Design review of the part built by this model. Coordinates are the model's own, in mm. Give positions to 0.01 mm unless a question says otherwise; leave off trailing zeros. Write each loop counter-clockwise with the first axis right and the second up, starting at its lowest first coordinate (ties: lowest second). Pieces come first, ordered by that corner, then holes. Notation, with made-up numbers: M 40,41.5 L 70,41.5 A20 ccw 70,61.5 Z; hole C 67,2 d9. An arc over 180 degrees is marked long. Use one line per item in the form item = value. Start each with the question number.
from build123d import *

# Parameters (mm, degrees)
SKETCH1_W           = 110
SKETCH1_H           = 85
BOSS_EXTRUDE1_DEPTH = 3
BOSS_EXTRUDE2_DEPTH = 1
SKETCH3_R           = 2.6
SKETCH3_R_2         = 1.5
CUT_EXTRUDE1_DEPTH  = 1
CUT_EXTRUDE2_REACH  = 6
SKETCH3_2_R         = 1.5
FILLET1_R           = 3
SKETCH15_R          = 1.75
CUT_EXTRUDE3_REACH  = 6
SKETCH17_R          = 3
SKETCH17_3_R        = 6
SKETCH17_3_R_2      = 3
CUT_EXTRUDE4_DEPTH  = 2
SKETCH18_W          = 20.4
SKETCH18_H          = 31.7
CUT_EXTRUDE5_DEPTH  = 5
SKETCH18_4_W        = 17
SKETCH18_4_H        = 5.15
BOSS_EXTRUDE3_DEPTH = 1.5
SKETCH19_R          = 1
CUT_EXTRUDE6_DEPTH  = 5
FILLET2_R           = 1


with BuildPart() as part:
    # Sketch1 → Boss-Extrude1 (new body)
    with BuildSketch(Plane(origin=(0, 0, 0), x_dir=(1, 0, 0), z_dir=(0, 1, 0))):
        with Locations((55, 42.5)):
            Rectangle(SKETCH1_W, SKETCH1_H)
    extrude(amount=BOSS_EXTRUDE1_DEPTH)

    # Sketch2 → Boss-Extrude2 (add)
    with BuildSketch(Plane.XZ):
        with BuildLine():
            ThreePointArc((100.9, -79.9), (102.071572875, -77.071572875), (104.9, -75.9))
            Line((104.9, -75.9), (104.9, -9.1))
            ThreePointArc((104.9, -9.1), (102.071572875, -7.928427125), (100.9, -5.1))
            Line((100.9, -5.1), (9.1, -5.1))
            ThreePointArc((9.1, -5.1), (7.928427125, -7.928427125), (5.1, -9.1))
            Line((5.1, -9.1), (5.1, -75.9))
            ThreePointArc((5.1, -75.9), (7.928427125, -77.071572875), (9.1, -79.9))
            Line((9.1, -79.9), (100.9, -79.9))
        make_face()
    extrude(amount=BOSS_EXTRUDE2_DEPTH)

    # Sketch3 → Cut-Extrude1 (cut)
    with BuildSketch(Plane(origin=(0, 3, 0), x_dir=(1, 0, 0), z_dir=(0, 1, 0))):
        with Locations((4, 81)):
            Circle(SKETCH3_R)
        with Locations((4, 81)):
            Circle(SKETCH3_R_2, mode=Mode.SUBTRACT)
        with Locations((106, 81)):
            Circle(SKETCH3_R)
        with Locations((106, 81)):
            Circle(SKETCH3_R_2, mode=Mode.SUBTRACT)
        with Locations((106, 4)):
            Circle(SKETCH3_R)
        with Locations((106, 4)):
            Circle(SKETCH3_R_2, mode=Mode.SUBTRACT)
        with Locations((4, 4)):
            Circle(SKETCH3_R)
        with Locations((4, 4)):
            Circle(SKETCH3_R_2, mode=Mode.SUBTRACT)
    extrude(amount=-CUT_EXTRUDE1_DEPTH, mode=Mode.SUBTRACT)

    # Sketch3<2> → Cut-Extrude2 (cut, up to next)
    with BuildSketch(Plane(origin=(0, 3, 0), x_dir=(1, 0, 0), z_dir=(0, 1, 0)), mode=Mode.PRIVATE) as cut_extrude2_sk1:
        with Locations((4, 81)):
            Circle(SKETCH3_2_R)
    cut_extrude2_tool1 = extrude(cut_extrude2_sk1.sketch, amount=-CUT_EXTRUDE2_REACH, mode=Mode.PRIVATE) & part.part
    add(cut_extrude2_tool1.solids().sort_by_distance((4, 3, -81))[0], mode=Mode.SUBTRACT)
    # Sketch3<2> → Cut-Extrude2 (cut, up to next)
    with BuildSketch(Plane(origin=(0, 3, 0), x_dir=(1, 0, 0), z_dir=(0, 1, 0)), mode=Mode.PRIVATE) as cut_extrude2_sk2:
        with Locations((106, 81)):
            Circle(SKETCH3_2_R)
    cut_extrude2_tool2 = extrude(cut_extrude2_sk2.sketch, amount=-CUT_EXTRUDE2_REACH, mode=Mode.PRIVATE) & part.part
    add(cut_extrude2_tool2.solids().sort_by_distance((106, 3, -81))[0], mode=Mode.SUBTRACT)
    # Sketch3<2> → Cut-Extrude2 (cut, up to next)
    with BuildSketch(Plane(origin=(0, 3, 0), x_dir=(1, 0, 0), z_dir=(0, 1, 0)), mode=Mode.PRIVATE) as cut_extrude2_sk3:
        with Locations((106, 4)):
            Circle(SKETCH3_2_R)
    cut_extrude2_tool3 = extrude(cut_extrude2_sk3.sketch, amount=-CUT_EXTRUDE2_REACH, mode=Mode.PRIVATE) & part.part
    add(cut_extrude2_tool3.solids().sort_by_distance((106, 3, -4))[0], mode=Mode.SUBTRACT)
    # Sketch3<2> → Cut-Extrude2 (cut, up to next)
    with BuildSketch(Plane(origin=(0, 3, 0), x_dir=(1, 0, 0), z_dir=(0, 1, 0)), mode=Mode.PRIVATE) as cut_extrude2_sk4:
        with Locations((4, 4)):
            Circle(SKETCH3_2_R)
    cut_extrude2_tool4 = extrude(cut_extrude2_sk4.sketch, amount=-CUT_EXTRUDE2_REACH, mode=Mode.PRIVATE) & part.part
    add(cut_extrude2_tool4.solids().sort_by_distance((4, 3, -4))[0], mode=Mode.SUBTRACT)

    # Fillet1
    fillet1_edges = [part.edges().sort_by_distance(p)[0] for p in [
        (0, 1.5, -85),
        (110, 1.5, -85),
        (110, 1.5, 0),
        (0, 1.5, 0),
    ]]
    fillet(fillet1_edges, radius=FILLET1_R)

    # Cut-Sweep3: sweep along a path in Sketch14
    with BuildLine(Plane.XZ) as cut_sweep3_path:
        Line((7.35, -5.1), (7.35, -3.35))
        Line((7.35, -3.35), (102.65, -3.35))
        Line((102.65, -3.35), (102.65, -5.1))
        ThreePointArc((102.65, -5.1), (103.309009742, -6.690990258), (104.9, -7.35))
        Line((104.9, -7.35), (106.65, -7.35))
        Line((106.65, -7.35), (106.65, -77.65))
        Line((106.65, -77.65), (104.9, -77.65))
        ThreePointArc((104.9, -77.65), (103.309009742, -78.309009742), (102.65, -79.9))
        Line((102.65, -79.9), (102.65, -81.65))
        Line((102.65, -81.65), (7.35, -81.65))
        Line((7.35, -81.65), (7.35, -79.9))
        ThreePointArc((7.35, -79.9), (6.690990258, -78.309009742), (5.1, -77.65))
        Line((5.1, -77.65), (3.35, -77.65))
        Line((3.35, -77.65), (3.35, -7.35))
        Line((3.35, -7.35), (5.1, -7.35))
        ThreePointArc((5.1, -7.35), (6.690990258, -6.690990258), (7.35, -5.1))
    # Sketch15 → Cut-Sweep3 (sweep, cut)
    with BuildSketch(Plane.XY.offset(-77.65)):
        with Locations((106.65, 0)):
            Circle(SKETCH15_R)
    sweep(path=cut_sweep3_path.line, transition=Transition.RIGHT, mode=Mode.SUBTRACT)

    # Sketch17 → Cut-Extrude3 (cut, up to next)
    with BuildSketch(Plane.XZ.offset(1), mode=Mode.PRIVATE) as cut_extrude3_sk1:
        with Locations((20, -20.1)):
            Circle(SKETCH17_R)
    cut_extrude3_tool1 = extrude(cut_extrude3_sk1.sketch, amount=-CUT_EXTRUDE3_REACH, mode=Mode.PRIVATE) & part.part
    add(cut_extrude3_tool1.solids().sort_by_distance((20, -1, -20.1))[0], mode=Mode.SUBTRACT)
    # Sketch17 → Cut-Extrude3 (cut, up to next)
    with BuildSketch(Plane.XZ.offset(1), mode=Mode.PRIVATE) as cut_extrude3_sk2:
        with Locations((90, -20.1)):
            Circle(SKETCH17_R)
    cut_extrude3_tool2 = extrude(cut_extrude3_sk2.sketch, amount=-CUT_EXTRUDE3_REACH, mode=Mode.PRIVATE) & part.part
    add(cut_extrude3_tool2.solids().sort_by_distance((90, -1, -20.1))[0], mode=Mode.SUBTRACT)

    # Sketch17<3> → Cut-Extrude4 (cut)
    with BuildSketch(Plane.XZ.offset(1)):
        with Locations((90, -20.1)):
            Circle(SKETCH17_3_R)
        with Locations((90, -20.1)):
            Circle(SKETCH17_3_R_2, mode=Mode.SUBTRACT)
        with Locations((20, -20.1)):
            Circle(SKETCH17_3_R)
        with Locations((20, -20.1)):
            Circle(SKETCH17_3_R_2, mode=Mode.SUBTRACT)
    extrude(amount=-CUT_EXTRUDE4_DEPTH, mode=Mode.SUBTRACT)

    # Sketch18 → Cut-Extrude5 (cut, through all)
    with BuildSketch(Plane.XZ.offset(1)):
        with Locations((55, -49.908642181)):
            Rectangle(SKETCH18_W, SKETCH18_H)
    extrude(amount=-CUT_EXTRUDE5_DEPTH, mode=Mode.SUBTRACT)

    # Sketch18<4> → Boss-Extrude3 (add)
    with BuildSketch(Plane.XZ.offset(1)):
        with Locations((55, -31.483642181)):
            Rectangle(SKETCH18_4_W, SKETCH18_4_H)
        with Locations((55, -68.333642181)):
            Rectangle(SKETCH18_4_W, SKETCH18_4_H)
    extrude(amount=BOSS_EXTRUDE3_DEPTH)

    # Sketch19 → Cut-Extrude6 (cut)
    with BuildSketch(Plane.XZ.offset(2.5)):
        with Locations((55, -31.908642181)):
            Circle(SKETCH19_R)
        with Locations((55, -67.908642181)):
            Circle(SKETCH19_R)
    extrude(amount=-CUT_EXTRUDE6_DEPTH, mode=Mode.SUBTRACT)

    # Fillet2
    fillet2_edges = [part.edges().sort_by_distance(p)[0] for p in [
        (63.5, -1.75, -28.908642181),
        (46.5, -1.75, -28.908642181),
        (46.5, -1.75, -70.908642181),
        (63.5, -1.75, -70.908642181),
    ]]
    fillet(fillet2_edges, radius=FILLET2_R)


solid = part.part
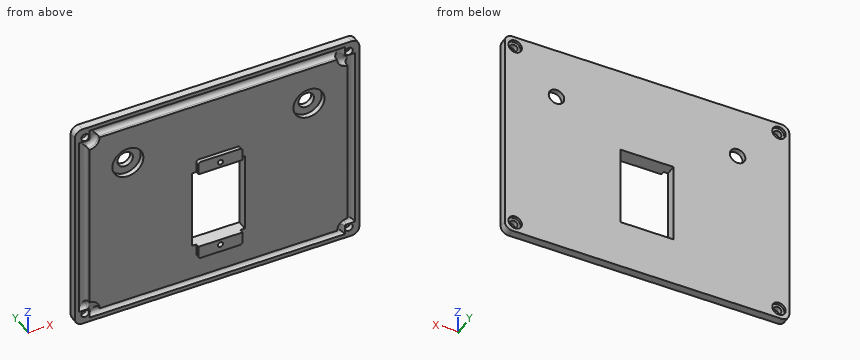
1. We need section B-B (z = -18.5). State the section outline as (x, y) points.
2. We need section A-A (z = -49). State the section outline as (x, y) points.
3. We need section C-C (x = 38.5). State the section outline as (y, z) points, and give its area (3 significant figures).
4. Clearance check with flat-ended pins moving along their axes: pin 1 Ø1.2 at (y, z) = (-2, -32.5) entering from +X; pin 2 Ø1.6 at (y, z) = (-2, -32.5) entering from -X; pin 3 Ø1.6 at (x, y) = (56, -1.5) entering from -Z; pin 4 Ø2.5 at (x, z) = (106, -4) entering from -Y. State where each tip first meets the part, or that it passes through.
5. To check wall thickness, follow L1, parallel to X at y = 2.45, z = -4; L2, parallel to Z at x = 4, y = 2.5; L3, parallel to Z at x = 26.5, y = 0.55. State the ranges of each line that lie inside material, in increasing order.
Answer block:
q1.outline = M 0,0 L 1.6,0 A1.75 cw 5.1,0 L 5.1,-1 L 14.22,-1 L 14.22,1 L 17.46,1 L 17.46,3 L 0,3 Z; M 22.54,1 L 25.78,1 L 25.78,-1 L 84.22,-1 L 84.22,1 L 87.46,1 L 87.46,3 L 22.54,3 Z; M 92.54,1 L 95.78,1 L 95.78,-1 L 104.9,-1 L 104.9,0 A1.75 cw 108.4,0 L 110,0 L 110,3 L 92.54,3 Z
q2.outline = M 0,0 L 1.6,0 A1.75 cw 5.1,0 L 5.1,-1 L 44.8,-1 L 44.8,3 L 0,3 Z; M 65.2,-1 L 104.9,-1 L 104.9,0 A1.75 cw 108.4,0 L 110,0 L 110,3 L 65.2,3 Z
q3.outline = M -1,-79.9 L 0,-79.9 A1.75 cw 0,-83.4 L 0,-85 L 3,-85 L 3,0 L 0,0 L 0,-1.6 A1.75 cw 0,-5.1 L -1,-5.1 Z
q3.area = 320 mm^2
q4.pin_1 = 63.5
q4.pin_2 = 46.5
q4.pin_3 = -79.9
q4.pin_4 = through
q5.L1 = 0 to 1.4, 6.6 to 103.4, 108.6 to 110
q5.L2 = -85 to -83.6, -78.4 to -6.6, -1.4 to 0
q5.L3 = -85 to -83.31, -79.99 to -5.01, -1.69 to 0
